Part model, mm, in its own coordinate system. A direction names the side the tool comes from. Round coordinates to 2 decimals unless told otherwise and drop trailing zeros. Write each loop counter-clockwise with the first axis right and the second up, starting at its lowest first coordinate (ties: lowest second). Pieces come first, ordered by that corner, then holes. Notation, with made-up numbers: M 50,44.25 L 107,44.25 A30 cw 107,79.25 Z; hole C 38,23 d3. An arc over 180 degrees is marked long. Use a Markdown table: item, result. Add a question column.
1) Which spindle directions (+Z, -Z, +X, -X, +Y, -Y) get a long thin tool onto all of the face, cutting with end or side? Do faces 4 (the face through (-158.44, 104.743, 149.09)), 5 (the face through (121.32, 86.89, 128.08)), 6 (the face through (-63.338, 52.492, 12.522)), 7 (the face through (-29, -48, 254)). Say none if no direction does.
2) Wall check: probe 1 along Y at (x, z) = (-89.5, 190); probe 2 along X at (y, z) = (185, 157); probe 3 along X at (y, z) = (56, 15.5). Give the ranges that are in metal, low to high.
3) Slice it at B-B on y = -42. Write the cut outline in (x, z), plus the area to 3 significant figures.
4) Slice it at C-C on x = -99.5. Write the cut outline in (y, z).
5) Two-plate mould, pull along Y, no slides. Class faces 1 (the face through (-145.562, 78, 113)), 2 (the face through (-16, 231.958, 107)), 3 (the face through (-9.835, 219.436, 140.61)): released by +Y, released by -Y, zero draft, split by the parting line, or undercut.
6) Slice it at A-A on z = 236. Write the cut outline in (x, y), plus the area to 3 significant figures.
7) Drop a flat-ended pin along its axis: P1, Ø10, axis at x = -36.5, y = -0.5, coming from the +Z side. Give the stop position or say it passes through.
```python
from build123d import *

# Parameters (mm, degrees)
F0_W      = 304.8
F0_H      = 304.8
F1_DEPTH  = 25.4
F3_DEPTH  = 254
F5_DEPTH  = 25.4
F7_DEPTH  = 25.4
F9_DEPTH  = 25.4
F11_DEPTH = 25.4
F13_DEPTH = 25.4
F15_DEPTH = 25.4


with BuildPart() as f1:
    # F0 (on Top) → F1 (new body)
    with BuildSketch(Plane.XY):
        with Locations((-18.562319, 79.558338)):
            Rectangle(F0_W, F0_H)
    extrude(amount=F1_DEPTH)

    # F2 (on face) → F3 (join)
    with BuildSketch(Plane.XY.offset(25.4)):
        Polygon((-145.562319, 231.958338), (-170.962319, 231.958338), (-170.962319, -72.841662), (108.437681, -72.841662), (108.437681, -47.441662), (-145.562319, -47.441662), (-145.562319, 206.558338), align=None)
        Polygon((133.837681, 231.958338), (-145.562319, 231.958338), (-145.562319, 206.558338), (108.437681, 206.558338), (108.437681, -47.441662), (108.437681, -72.841662), (133.837681, -72.841662), align=None)
    extrude(amount=F3_DEPTH)

    # F4 (on face) → F5 (cut)
    with BuildSketch(Plane.XY.offset(279.4)):
        Polygon((-145.562319, 212.908338), (-145.562319, 206.558338), (108.437681, 206.558338), (108.437681, -47.441662), (108.437681, -53.791662), (114.787681, -53.791662), (114.787681, 212.908338), align=None)
        Polygon((-145.562319, -47.441662), (-145.562319, 206.558338), (-145.562319, 212.908338), (-151.912319, 212.908338), (-151.912319, -53.791662), (108.437681, -53.791662), (108.437681, -47.441662), align=None)
    extrude(amount=-F5_DEPTH, mode=Mode.SUBTRACT)

    # F6 (on face) → F7 (cut)
    with BuildSketch(Plane.XZ.offset(72.841662)):
        with BuildLine():
            ThreePointArc((6.837681, 152.4), (-0.601807, 170.360512), (-18.562319, 177.8))
            ThreePointArc((-18.562319, 177.8), (-36.522831, 134.439488), (6.837681, 152.4))
        make_face()
    extrude(amount=-F7_DEPTH, mode=Mode.SUBTRACT)

    # F8 (on face) → F9 (cut)
    with BuildSketch(Plane.YZ.offset(133.837681)):
        Polygon((86.032008, 181.00603), (79.558338, 178.996087), (58.021625, 172.309378), (51.547955, 143.703348), (73.084668, 123.79397), (101.095051, 132.490622), (107.568721, 161.096652), align=None)
    extrude(amount=-F9_DEPTH, mode=Mode.SUBTRACT)

    # F10 (on face) → F11 (cut)
    with BuildSketch(Plane(origin=(0, 231.958338, 0), x_dir=(-1, 0, 0), z_dir=(0, 1, 0))):
        Polygon((35.435384, 176.389852), (18.562319, 168.564909), (-10.650035, 155.017578), (30.901607, 125.792571), align=None)
    extrude(amount=-F11_DEPTH, mode=Mode.SUBTRACT)

    # F12 (on face) → F13 (cut)
    with BuildSketch(Plane(origin=(0, 0, 0), x_dir=(1, 0, 0), z_dir=(0, 0, -1))):
        Polygon((17.358706, -43.637314), (-18.562319, -79.558338), (-54.483343, -43.637314), (-72.443855, -61.597826), (-36.522831, -97.51885), (-72.443855, -133.439875), (-54.483343, -151.400387), (-18.562319, -115.479363), (17.358706, -151.400387), (35.319218, -133.439875), (-0.601807, -97.51885), (35.319218, -61.597826), align=None)
    extrude(amount=-F13_DEPTH, mode=Mode.SUBTRACT)

    # F14 (on face) → F15 (cut)
    with BuildSketch(Plane(origin=(-170.962319, 0, 0), x_dir=(0, -1, 0), z_dir=(-1, 0, 0))):
        Polygon((-74.14409, 183.325761), (-79.558338, 180.676894), (-107.29739, 167.105841), (-102.116263, 130.562949), (-65.76085, 124.198119), (-48.473097, 156.80733), align=None)
    extrude(amount=-F15_DEPTH, mode=Mode.SUBTRACT)


solid = f1.part
```
Entries:
| question | item | result |
|---|---|---|
| 1 | face 4 | -X |
| 1 | face 5 | +X |
| 1 | face 6 | +Z, -Z |
| 1 | face 7 | +Z |
| 2 | probe 1 | y = -72.84 to -47.44, 206.56 to 231.96 |
| 2 | probe 2 | x = -170.96 to -145.56, 108.44 to 133.84 |
| 2 | probe 3 | x = -170.96 to -66.85, -42.12 to 5, 29.72 to 133.84 |
| 3 | outline | M -170.96,0 L 133.84,0 L 133.84,279.4 L 114.79,279.4 L 114.79,254 L 108.44,254 L 108.44,25.4 L -145.56,25.4 L -145.56,254 L -151.91,254 L -151.91,279.4 L -170.96,279.4 Z |
| 3 | area | 20,300 mm^2 |
| 4 | outline | M -72.84,0 L 231.96,0 L 231.96,279.4 L 212.91,279.4 L 212.91,254 L 206.56,254 L 206.56,25.4 L -47.44,25.4 L -47.44,254 L -53.79,254 L -53.79,279.4 L -72.84,279.4 Z |
| 5 | face 1 | undercut |
| 5 | face 2 | released by +Y |
| 5 | face 3 | zero draft |
| 6 | outline | M -170.96,-72.84 L 133.84,-72.84 L 133.84,231.96 L -170.96,231.96 Z; hole M -145.56,-47.44 L 108.44,-47.44 L 108.44,206.56 L -145.56,206.56 Z |
| 6 | area | 28,400 mm^2 |
| 7 | P1 | stops at z = 25.4 |
